Autodesk Inventor part; units mm, degrees
ref_plane "YZ Plane" through (0, 0, 0) normal (1, 0, 0) x (0, 1, 0)
ref_plane "XZ Plane" through (0, 0, 0) normal (0, 1, 0) x (-1, 0, 0)
ref_plane "XY Plane" through (0, 0, 0) normal (0, 0, 1) x (1, 0, 0)
sketch "Sketch1" plane through (0, 0, 0) normal (1, 0, 0) x (0, 1, 0)
  line L0 (0, 0) -> (0, 36)
  line L1 (0, 36) -> (6, 36)
  line L2 (6, 36) -> (6, 6)
  line L3 (6, 6) -> (56, 6)
  line L4 (56, 6) -> (56, 0)
  line L5 (56, 0) -> (0, 0)
  dimension "d0" = 36
  dimension "d1" = 6
  dimension "d2" = 30
  dimension "d3" = 50
  dimension "d4" = 6
  dimension "d5" = 56
extrude "Extrusion1" add sketch "Sketch1" against normal blind 60
sketch "Sketch2" plane through (0, 6, 36) normal (0, 1, 0) x (1, 0, 0)
  circle A0 centre (-52, 15) radius 3.25
  circle A1 centre (-32, 15) radius 3.25
  line L0 (0, 0) -> (-60, 0)
  line L1 (0, 30) -> (0, 0)
  line L2 (-60, 0) -> (-60, 30)
  line L3 (-60, 30) -> (-20.277, 30) construction
  point P0 (0, 36)
  point P1 (-5.4498, 30)
  dimension "d8" = 6.5
  dimension "d9" = 6.5
  dimension "d10" = 20
  dimension "d11" = 15
  dimension "d12" = 15
  dimension "d13" = 32
sketch "Sketch3" plane through (0, 6, 6) normal (0, 0, 1) x (1, 0, 0)
  circle A0 centre (-52, 30) radius 3.25
  line L0 (-60, 0) -> (-60, 50)
  line L1 (0, 50) -> (-60, 50)
  circle A1 centre (-32, 30) radius 3.25
  point P0 (0, -6)
  dimension "d14" = 6.5
  dimension "d15" = 8
  dimension "d16" = 20
  dimension "d17" = 6.5
  dimension "d18" = 20
  dimension "d27" = 50
extrude "Extrusion2" cut sketch "Sketch3" against normal blind 6
extrude "Extrusion3" cut sketch "Sketch2" against normal blind 6
sketch "Sketch4" plane through (0, 6, 6) normal (0, 0, 1) x (1, 0, 0)
  circle A0 centre (-10, 35) radius 6.35
  line L0 (0, 50) -> (0, 0)
  line L1 (0, 50) -> (-60, 50)
  line L2 (-60, 0) -> (-60, 50)
  point P0 (0, -6)
  point P1 (0, 25)
  dimension "d23" = 12.7
  dimension "d28" = 15
  dimension "d29" = 50
extrude "Extrusion4" cut sketch "Sketch4" against normal blind 6
properties part number "Base_Connector1"
Verification items for the finished model (mm, model axes). A direction names the side the tool comes from. Coordinates: 2 decimals unless noted, no trailing zeros. Order: outer loops, then holes, each group sorted by start corner. A loop starts at its lowest first (then second) coordinate and runs counter-clockwise, first axis right, second up.
1. Sectioned sample at D-D, the plane x = -6. Record the cut outline in (y, z), and give its area (3 significant figures).
Results found:
outline: (0, 0) - (36.07, 0) - (36.07, 6) - (6, 6) - (6, 36) - (0, 36) - close; (45.93, 0) - (56, 0) - (56, 6) - (45.93, 6) - close
area: 457 mm2
2. Sectioned sample at B-B, the plane x = -32. Record the cut outline in (y, z), and give its area (3 significant figures).
Results found:
outline: (0, 0) - (32.75, 0) - (32.75, 6) - (6, 6) - (6, 17.75) - (0, 17.75) - close; (0, 24.25) - (6, 24.25) - (6, 36) - (0, 36) - close; (39.25, 0) - (56, 0) - (56, 6) - (39.25, 6) - close
area: 438 mm2
3. Set-up check for faces 4 (the face through (-30, 6, 25)), 5 (the face through (-60, 17, 5)): record each of +Z, -Z, +X, -X, +Y, -Y from which the full face is reachable in a straight line by a thin tool's end or side.
Results found:
face 4: +Z, +X, -X, +Y
face 5: +Z, -Z, -X, +Y, -Y
4. Sectioned sample at A-A, the plane y = 41. Record the cut outline in (x, z), and give its area (3 significant figures).
Results found:
outline: (-60, 0) - (-16.35, 0) - (-16.35, 6) - (-60, 6) - close; (-3.65, 0) - (0, 0) - (0, 6) - (-3.65, 6) - close
area: 284 mm2
5. Sectioned sample at C-C, the plane z = 21. Record the cut outline in (x, y), and give its area (3 significant figures).
Results found:
outline: (-60, 0) - (-55.25, 0) - (-55.25, 6) - (-60, 6) - close; (-48.75, 0) - (-35.25, 0) - (-35.25, 6) - (-48.75, 6) - close; (-28.75, 0) - (0, 0) - (0, 6) - (-28.75, 6) - close
area: 282 mm2
6. Release check for a two-part mould opening along X. For faces 1 (the face through (-50.5, 33.117, 3.042)), 2 (the face through (-30, 0, 18)), 3 (the face through (0, 17, 5)) record: +X half, -X half, draft (parallel to the pull), parting line (faces both ways), or undercut.
Results found:
face 1: undercut
face 2: draft
face 3: +X half
7. Scan lines: line 1 (X direction, y = 1, z = 21); line 2 (Y direction, x = -32, z = 2.7); line 3 (Y direction, x = -10, z = 2). Record each from-to range of solid material in increasing order.
Results found:
line 1: x = -60 to -55.25, -48.75 to -35.25, -28.75 to 0
line 2: y = 0 to 32.75, 39.25 to 56
line 3: y = 0 to 34.65, 47.35 to 56
8. Go/stop test with flat-tipped pins: pin 1 Ø4 at (x, y) = (-41, 49.5) entering from +Z; pin 2 Ø4 at (x, z) = (-52, 21) entering from -Y; pin 3 Ø1 at (x, z) = (-38.5, 31.5) entering from +Y. Record where each tip stops, or that it passes through.
Results found:
pin 1: stops at z = 6
pin 2: passes through
pin 3: stops at y = 6
